```python
from build123d import *

# Parameters (mm, degrees)
BOSS_EXTRU_1_DEPTH      = 3
ESQUISSE3_W             = 33.6
ESQUISSE3_H             = 3
BOSS_EXTRU_2_DEPTH      = 24
ESQUISSE4_W             = 5
ESQUISSE4_H             = 5
ESQUISSE4_R             = 1.25
BOSS_EXTRU_3_DEPTH      = 2.8
BOSS_EXTRU_4_START      = -2.8
ESQUISSE5_W             = 5
ESQUISSE5_H             = 5
ESQUISSE5_R             = 1.25
BOSS_EXTRU_4_DEPTH      = 2.8
ESQUISSE4_2_W           = 5
ESQUISSE4_2_H           = 5
ESQUISSE4_2_R           = 1.25
BOSS_EXTRU_5_DEPTH      = 4.8
ESQUISSE6_W             = 5
ESQUISSE6_H             = 40
ESQUISSE6_R             = 1.75
BOSS_EXTRU_6_DEPTH      = 9
CONG_3_R                = 10
CONG_4_R                = 1
CONG_1_R                = 1.45
CONG_2_R                = 1
ENL_V_MAT_EXTRU_1_REACH = 65.655
ESQUISSE6_3_R           = 1.75


with BuildPart() as part:
    # Esquisse1 → Boss.-Extru.1 (new body)
    with BuildSketch(Plane.XY):
        Polygon((-15, -20), (15, -20), (15, 20), (-15, 20), (-48.6, 20), (-48.6, -31), (-15, -31), align=None)
    extrude(amount=BOSS_EXTRU_1_DEPTH)

    # Esquisse3 → Boss.-Extru.2 (add)
    with BuildSketch(Plane(origin=(0, 0, 0), x_dir=(-1, 0, 0), z_dir=(0, 0, -1))):
        with Locations((31.8, -29.5)):
            Rectangle(ESQUISSE3_W, ESQUISSE3_H)
        with Locations((31.8, 18.5)):
            Rectangle(ESQUISSE3_W, ESQUISSE3_H)
    extrude(amount=BOSS_EXTRU_2_DEPTH)

    # Esquisse4 → Boss.-Extru.3 (add)
    # profile 1 of 4: a face of its own
    with BuildSketch(Plane.ZY.offset(48.6)):
        with Locations((-21.5, -25.5)):
            Rectangle(ESQUISSE4_W, ESQUISSE4_H)
        with Locations(Location((-21, -25, 0), (0, 0, 270))):
            Circle(ESQUISSE4_R, mode=Mode.SUBTRACT)
    # profile 2 of 4: a face of its own
    with BuildSketch(Plane.ZY.offset(48.6)):
        with Locations((-2.5, -25.5)):
            Rectangle(ESQUISSE4_W, ESQUISSE4_H)
        with Locations(Location((-3, -25, 0), (0, 0, 90))):
            Circle(ESQUISSE4_R, mode=Mode.SUBTRACT)
    # profile 3 of 4: a face of its own
    with BuildSketch(Plane.ZY.offset(48.6)):
        with Locations((-2.5, 14.5)):
            Rectangle(ESQUISSE4_W, ESQUISSE4_H)
        with Locations(Location((-3, 14, 0), (0, 0, 270))):
            Circle(ESQUISSE4_R, mode=Mode.SUBTRACT)
    # profile 4 of 4: a face of its own
    with BuildSketch(Plane.ZY.offset(48.6)):
        with Locations((-21.5, 14.5)):
            Rectangle(ESQUISSE4_W, ESQUISSE4_H)
        with Locations(Location((-21, 14, 0), (0, 0, 90))):
            Circle(ESQUISSE4_R, mode=Mode.SUBTRACT)
    extrude(amount=-BOSS_EXTRU_3_DEPTH)

    # Esquisse5 → Boss.-Extru.4 (add)
    # profile 1 of 3: a face of its own
    with BuildSketch(Plane(origin=(-15, 0, 0), x_dir=(0, 0, -1), z_dir=(1, 0, 0)).offset(BOSS_EXTRU_4_START)):
        with Locations((2.5, -25.5)):
            Rectangle(ESQUISSE5_W, ESQUISSE5_H)
        with Locations(Location((3, -25, 0), (0, 0, 90))):
            Circle(ESQUISSE5_R, mode=Mode.SUBTRACT)
    # profile 2 of 3: a face of its own
    with BuildSketch(Plane(origin=(-15, 0, 0), x_dir=(0, 0, -1), z_dir=(1, 0, 0)).offset(BOSS_EXTRU_4_START)):
        with Locations((2.5, 14.5)):
            Rectangle(ESQUISSE5_W, ESQUISSE5_H)
        with Locations(Location((3, 14, 0), (0, 0, 270))):
            Circle(ESQUISSE5_R, mode=Mode.SUBTRACT)
    # profile 3 of 3: a face of its own
    with BuildSketch(Plane(origin=(-15, 0, 0), x_dir=(0, 0, -1), z_dir=(1, 0, 0)).offset(BOSS_EXTRU_4_START)):
        with Locations((2.5, 3.3)):
            Rectangle(ESQUISSE5_W, ESQUISSE5_H)
        with Locations((3, 3.3)):
            Circle(ESQUISSE5_R, mode=Mode.SUBTRACT)
    extrude(amount=BOSS_EXTRU_4_DEPTH)

    # Esquisse4<2> → Boss.-Extru.5 (add)
    # profile 1 of 2: a face of its own
    with BuildSketch(Plane.ZY.offset(48.6)):
        with Locations((-21.5, -25.5)):
            Rectangle(ESQUISSE4_2_W, ESQUISSE4_2_H)
        with Locations(Location((-21, -25, 0), (0, 0, 270))):
            Circle(ESQUISSE4_2_R, mode=Mode.SUBTRACT)
    # profile 2 of 2: a face of its own
    with BuildSketch(Plane.ZY.offset(48.6)):
        with Locations((-2.5, -25.5)):
            Rectangle(ESQUISSE4_2_W, ESQUISSE4_2_H)
        with Locations(Location((-3, -25, 0), (0, 0, 270))):
            Circle(ESQUISSE4_2_R, mode=Mode.SUBTRACT)
    extrude(amount=-BOSS_EXTRU_5_DEPTH)

    # Esquisse6 → Boss.-Extru.6 (add)
    # profile 1 of 2: a face of its own
    with BuildSketch(Plane.XY.offset(3)):
        with Locations((12.5, 0)):
            Rectangle(ESQUISSE6_W, ESQUISSE6_H)
        with Locations(Location((12.5, -15, 0), (0, 0, 180))):
            Circle(ESQUISSE6_R, mode=Mode.SUBTRACT)
        with Locations((12.5, 15)):
            Circle(ESQUISSE6_R, mode=Mode.SUBTRACT)
    # profile 2 of 2: a face of its own
    with BuildSketch(Plane.XY.offset(3)):
        with Locations((-12.5, 0)):
            Rectangle(ESQUISSE6_W, ESQUISSE6_H)
        with Locations((-12.5, -15)):
            Circle(ESQUISSE6_R, mode=Mode.SUBTRACT)
        with Locations((-12.5, 15)):
            Circle(ESQUISSE6_R, mode=Mode.SUBTRACT)
    extrude(amount=BOSS_EXTRU_6_DEPTH)

    # Congé3
    # the kernel refuses this fillet: 10 mm, written as the material it adds along each edge
    with BuildSketch(Plane(origin=(-15, 20, 3), x_dir=(-1, 0, 0), z_dir=(0, -1, 0))) as cong_3_piece_1:
        with BuildLine():
            CenterArc((9.949874371, -10), CONG_3_R, 90, 84.260829523)
            Line((0, -9), (0, 0))
            Line((0, 0), (9.949874371, 0))
        make_face()
    extrude(amount=40)

    # Congé4
    # the kernel refuses this fillet: 1 mm, written as the material it adds along each edge
    with BuildSketch(Plane(origin=(-15, -20, 0), x_dir=(1, 0, 0), z_dir=(0, 0, 1))) as cong_4_piece_1:
        with BuildLine():
            CenterArc((CONG_4_R, -CONG_4_R), CONG_4_R, 90, 90)
            Line((0, -CONG_4_R), (0, 0))
            Line((0, 0), (CONG_4_R, 0))
        make_face()
    extrude(amount=3)
    with BuildSketch(Plane(origin=(-15, 0.8, 0), x_dir=(1, 0, 0), z_dir=(0, 1, 0))) as cong_4_piece_2:
        with BuildLine():
            CenterArc((CONG_4_R, CONG_4_R), CONG_4_R, 180, 90)
            Line((0, CONG_4_R), (0, 0))
            Line((0, 0), (CONG_4_R, 0))
        make_face()
    extrude(amount=5)
    with BuildSketch(Plane(origin=(-15, 12, 0), x_dir=(1, 0, 0), z_dir=(0, 1, 0))) as cong_4_piece_3:
        with BuildLine():
            CenterArc((CONG_4_R, CONG_4_R), CONG_4_R, 180, 90)
            Line((0, CONG_4_R), (0, 0))
            Line((0, 0), (CONG_4_R, 0))
        make_face()
    extrude(amount=8)

    # Congé1
    cong_1_edges = [part.edges().sort_by_distance(p)[0] for p in [
        (-16.4, 12, -5),
        (-16.4, 5.8, -5),
        (-16.4, 0.8, -5),
        (-16.4, -23, -5),
        (-16.4, -28, -5),
        (-46.2, -23, -19),
        (-46.2, -28, -19),
        (-46.2, -28, -5),
        (-46.2, -23, -5),
        (-47.2, 12, -5),
        (15, 0, 0),
        (-47.2, 12, -19),
    ]]
    fillet(cong_1_edges, radius=CONG_1_R)

    # Congé2
    cong_2_edges = [part.edges().sort_by_distance(p)[0] for p in [
        (-47.2, 12, -24),
        (-16.4, -23, 0),
        (-15.9, 12, 0),
        (-15.9, 0.8, 0),
        (-15.9, 5.8, 0),
        (-46.2, -23, -24),
    ]]
    fillet(cong_2_edges, radius=CONG_2_R)

    # Esquisse6<3> → Enlèv. mat.-Extru.1 (cut, up to next)
    with BuildSketch(Plane.XY.offset(3), mode=Mode.PRIVATE) as enl_v_mat_extru_1_sk1:
        with Locations(Location((-12.5, 15, 0), (0, 0, 211.002719134))):
            Circle(ESQUISSE6_3_R)
    enl_v_mat_extru_1_tool1 = extrude(enl_v_mat_extru_1_sk1.sketch, amount=-ENL_V_MAT_EXTRU_1_REACH, mode=Mode.PRIVATE) & part.part
    # Esquisse6<3> → Enlèv. mat.-Extru.1 (cut, up to next)
    with BuildSketch(Plane.XY.offset(3), mode=Mode.PRIVATE) as enl_v_mat_extru_1_sk2:
        with Locations(Location((-12.5, -15, 0), (0, 0, 180))):
            Circle(ESQUISSE6_3_R)
    enl_v_mat_extru_1_tool2 = extrude(enl_v_mat_extru_1_sk2.sketch, amount=-ENL_V_MAT_EXTRU_1_REACH, mode=Mode.PRIVATE) & part.part
    # Esquisse6<3> → Enlèv. mat.-Extru.1 (cut, up to next)
    with BuildSketch(Plane.XY.offset(3), mode=Mode.PRIVATE) as enl_v_mat_extru_1_sk3:
        with Locations(Location((12.5, -15, 0), (0, 0, 53.130102354))):
            Circle(ESQUISSE6_3_R)
    enl_v_mat_extru_1_tool3 = extrude(enl_v_mat_extru_1_sk3.sketch, amount=-ENL_V_MAT_EXTRU_1_REACH, mode=Mode.PRIVATE) & part.part
    # Esquisse6<3> → Enlèv. mat.-Extru.1 (cut, up to next)
    with BuildSketch(Plane.XY.offset(3), mode=Mode.PRIVATE) as enl_v_mat_extru_1_sk4:
        with Locations(Location((12.5, 15, 0), (0, 0, 306.869897646))):
            Circle(ESQUISSE6_3_R)
    enl_v_mat_extru_1_tool4 = extrude(enl_v_mat_extru_1_sk4.sketch, amount=-ENL_V_MAT_EXTRU_1_REACH, mode=Mode.PRIVATE) & part.part
    add(enl_v_mat_extru_1_tool1.solids().sort_by_distance((-12.5, 15, 3))[0], mode=Mode.SUBTRACT)
    add(enl_v_mat_extru_1_tool2.solids().sort_by_distance((-12.5, -15, 3))[0], mode=Mode.SUBTRACT)
    add(enl_v_mat_extru_1_tool3.solids().sort_by_distance((12.5, -15, 3))[0], mode=Mode.SUBTRACT)
    add(enl_v_mat_extru_1_tool4.solids().sort_by_distance((12.5, 15, 3))[0], mode=Mode.SUBTRACT)


solid = part.part
```
Design review of the part built by this model. Coordinates are the model's own, in mm. A direction names the side the tool comes from. Give positions to 0.01 mm unless a question says otherwise; leave off trailing zeros. Loops run counter-clockwise (first coordinate to the right, second up) from the corner with the lowest first, then second, coordinate; pieces in that order, holes last. Notation, with made-up numbers: (58.25, 13.25) -> (68.25, 13.25) arc R25 cw to (68.25, 52.25) -> close; hole circle Ø9 at (-24, 38). An arc over 180 degrees is marked (long way). One line per item, written item: value.
Q1. We need section D-D on z = 10. Give the boundary of the cut face in (x, y).
Numbers:
outline: (-15.41, -20) -> (-10, -20) -> (-10, 20) -> (-15.41, 20) -> close; (10, -20) -> (15, -20) -> (15, 20) -> (10, 20) -> close; hole circle Ø3.5 at (-12.5, -15); hole circle Ø3.5 at (-12.5, 15); hole circle Ø3.5 at (12.5, -15); hole circle Ø3.5 at (12.5, 15)
Q2. For L1, parallel to Y at x = -12.5, z = 6; L2, parallel to Z at x = -47, y = 14; L3, parallel to X at y = -15, z = 6, list the stretches that pass through material, from the lowest coordinate up.
Numbers:
L1: y = -20 to -16.75, -13.25 to 13.25, 16.75 to 20
L2: z = -24 to -22.25, -19.75 to -19, -5 to -4.25, -1.75 to 3
L3: x = -17.81 to -14.25, -10.75 to -10, 10 to 10.75, 14.25 to 15
Q3. For pin 1 Ø5.5 at (y, z) = (14, -3.5) entering from +X; pin 2 Ø8 at (y, z) = (8, -15.5) entering from -X; pin 3 Ø4.5 at (y, z) = (7.5, 6.5) entering from -X; pin 4 Ø5 at (x, y) = (6.5, -7) entering from +Z, all flat-tipped, find the tip position at first contact; note any pin that passes through.
Numbers:
pin 1: stops at x = -14.97
pin 2: passes through
pin 3: stops at x = -20.11
pin 4: stops at z = 3
Q4. We need section A-A on z = -14.5. Give the boundary of the cut face in (x, y), and give its area (3 significant figures).
Numbers:
outline: (-48.6, -31) -> (-15, -31) -> (-15, -28) -> (-48.6, -28) -> close; (-48.6, 17) -> (-15, 17) -> (-15, 20) -> (-48.6, 20) -> close
area: 202 mm^2
Q5. We need section B-B on y = 3.3. Give the boundary of the cut face in (x, z).
Numbers:
outline: (-48.6, 0) -> (-17.8, 0) -> (-17.8, -1.75) -> (-15, -1.75) -> (-15, -1) arc R1 cw to (-14, 0) -> (13.55, 0) arc R1.45 ccw to (15, 1.45) -> (15, 12) -> (10, 12) -> (10, 3) -> (-10, 3) -> (-10, 12) -> (-15, 12) arc R10 cw to (-24.95, 3) -> (-48.6, 3) -> close; (-17.8, -5) -> (-15, -5) -> (-15, -4.25) -> (-17.8, -4.25) -> close
Q6. Machinability: for faces 4 (the flat face through (-47, 15, -19)), 5 (the flat face through (-16, 3, -5)), 6 (the flat face through (-2, -20, 2)), which of the approach directions +Z, -Z, +X, -X, +Y, -Y give a long, thin tool a straight path to every point of the face, cutting with its end or side? Answer none if there is none.
Numbers:
face 4: +X, -X
face 5: -Z, +X, -X
face 6: +Z, +X, -Y
Q7. We need section C-C on x = -33. Give the boundary of the cut face in (y, z), and give its area (3 significant figures).
Numbers:
outline: (-31, -24) -> (-28, -24) -> (-28, 0) -> (17, 0) -> (17, -24) -> (20, -24) -> (20, 3) -> (-31, 3) -> close
area: 297 mm^2
Q8. Draft analysis for pull direction X (two halves, no side actions). For faces 1 (the flat face through (-43.8, -26, -22)), 2 (the cylindrical face through (-16.38, 1.24, -4.59)), 3 (the flat face through (-17.8, 15, -2)), state which applies: pulls with the +X half, pulls with the -X half, needs draft (parallel to the pull), parting line crosses it, or undercut.
Numbers:
face 1: pulls with the +X half
face 2: needs draft
face 3: undercut
